```python
from build123d import *

# Parameters (mm, degrees)
BOSS_EXTRUDE1_DEPTH = 52.5
FILLET1_R           = 1


with BuildPart() as part:
    # Sketch1 → Boss-Extrude1 (new, symmetric)
    with BuildSketch(Plane.XY):
        Polygon((5, -55), (5, -60), (10, -55), (10, 55), (0, 55), (0, -55), align=None)
    extrude(amount=BOSS_EXTRUDE1_DEPTH, both=True)

    # Fillet1
    fillet1_edges = [part.edges().sort_by_distance(p)[0] for p in [
        (10, -55, 0),
        (0, -55, 0),
        (0, 55, 0),
        (10, 55, 0),
    ]]
    fillet(fillet1_edges, radius=FILLET1_R)


solid = part.part
```
Could you check a few things on this model? Use its own coordinates, in mm. A direction names the side the tool comes from. Round coordinates to 2 decimals unless told otherwise and drop trailing zeros. Write each loop counter-clockwise with the first axis right and the second up, starting at its lowest first coordinate (ties: lowest second). Pieces come first, ordered by that corner, then holes.
(1) Suppose I cut it at A-A on z = -14. Write out the boundary of the cut face in (x, y).
Findings below:
outline: (0, -54) arc R1 ccw to (1, -55) - (5, -55) - (5, -60) - (9.71, -55.29) arc R1 ccw to (10, -54.59) - (10, 54) arc R1 ccw to (9, 55) - (1, 55) arc R1 ccw to (0, 54) - close
(2) For pin 1 (5.5 mm diameter, centred on y = -58, z = -22.5, fed in from -X); pin 2 (2 mm diameter, centred on x = 2.5, z = -10.5, fed in from -Y), each with a flat end and sliding along its axis, tell me the tip position at first contact or that it passes through.
Findings below:
pin 1: stops at x = 5
pin 2: stops at y = -55
(3) If I drill on probe 1 along Y at (x, z) = (1.5, -22.5); probe 2 along Y at (x, z) = (6.5, -7), over which ranges is the centre line in solid material (lowest first)?
Findings below:
probe 1: y = -55 to 55
probe 2: y = -58.5 to 55
(4) Which directions (+Z, -Z, +X, -X, +Y, -Y) give clear straight access to the entire face, cutting with the end or side of a thin tool? Please do faces 1 (the face through (5, -57, 1)), 2 (the face through (5, -2, 52.5)).
Findings below:
face 1: +Z, -Z, -X, -Y
face 2: +Z, +X, -X, +Y, -Y
(5) Suppose I cut it at B-B on x = 3.25. Write out the boundary of the cut face in (y, z).
Findings below:
outline: (-55, -52.5) - (55, -52.5) - (55, 52.5) - (-55, 52.5) - close
